Autodesk Inventor part; units mm, degrees
ref_plane "YZ Plane" through (0, 0, 0) normal (1, 0, 0) x (0, 1, 0)
ref_plane "XZ Plane" through (0, 0, 0) normal (0, 1, 0) x (-1, 0, 0)
ref_plane "XY Plane" through (0, 0, 0) normal (0, 0, 1) x (1, 0, 0)
sketch "Sketch1" plane through (0, 0, 0) normal (0, 0, 1) x (1, 0, 0)
  line L0 (-42.5, 5) -> (42.5, 5)
  line L1 (42.5, 5) -> (42.5, -5)
  line L2 (42.5, -5) -> (-42.5, -5)
  line L3 (-42.5, -5) -> (-42.5, 5)
  line L4 (-42.5, 5) -> (42.5, -5) construction
  line L5 (42.5, 5) -> (-42.5, -5) construction
  point P0 (0, 0)
  dimension "d0" = 85
  dimension "d1" = 10
extrude "Extrusion1" add sketch "Sketch1" along normal blind 0.5
sketch "Sketch2" plane through (0, 0, 0.5) normal (0, 0, 1) x (1, 0, 0)
  line L0 (-36.5, 2.5) -> (-31.5, 2.5)
  line L1 (-31.5, 2.5) -> (-31.5, -2.5)
  line L2 (-31.5, -2.5) -> (-36.5, -2.5)
  line L3 (-36.5, -2.5) -> (-36.5, 2.5)
  line L4 (-36.5, 2.5) -> (-31.5, -2.5) construction
  line L5 (-31.5, 2.5) -> (-36.5, -2.5) construction
  line L6 (-42.5, 5) -> (-42.5, -5)
  point P0 (0, 0)
  point P1 (-34, 0)
  point P2 (-34, 0)
  point P3 (-42.5, 0)
  dimension "d4" = 5
  dimension "d5" = 5
  dimension "d6" = 6
extrude "Extrusion2" add sketch "Sketch2" along normal blind 1.6
sketch "Sketch3" plane through (0, 0, 2.1) normal (0, 0, 1) x (1, 0, 0)
  line L0 (-31.5, 2.5) -> (-36.5, 2.5)
  line L1 (-36.5, 2.5) -> (-36.5, -2.5)
  line L2 (-36.5, -2.5) -> (-31.5, -2.5)
  line L3 (-31.5, -2.5) -> (-31.5, 2.5)
  circle A0 centre (-34, 0) radius 2.05
  point P0 (0, 0)
  point P1 (-31.5, 0)
  point P2 (-34, 2.5)
  dimension "d9" = 4.1
extrude "Extrusion3" cut sketch "Sketch3" against normal blind 0.1 contours A0
pattern_linear "Rectangular Pattern1" count 5 spacing 17 along (1, 0, 0) of "Extrusion3", "Extrusion2"
properties part number "LED Strip 5050 x 5"
Part model, mm, in its own coordinate system. A direction names the side the tool comes from. Give positions to 0.01 mm unless a question says otherwise; leave off trailing zeros. Write each loop counter-clockwise with the first axis right and the second up, starting at its lowest first coordinate (ties: lowest second). Pieces come first, ordered by that corner, then holes. Notation, with made-up numbers: (6.5, 5) -> (58.5, 5) arc R13 ccw to (58.5, 13) -> close; hole circle Ø2 at (62.5, 51.25). An arc over 180 degrees is marked (long way). Put each result on its own line as item: value. Start each with the question number.
Item 1: Cut at C-C (x = 4). List the corners of the cut face in (y, z).
Item 2: Pull direction X, two halves, no side cores. Call faces 1 (the face through (36.5, 0, 1)), 2 (the face through (-1, 0, 0)), 3 (the face through (0, 0, 2)): pulls with the +X half, pulls with the -X half, needs draft (parallel to the pull), parting line crosses it, or undercut.
Item 3: Which spindle directions (+Z, -Z, +X, -X, +Y, -Y) get a long thin tool onto all of the face, cutting with end or side? Do faces 4 (the face through (19.5, 0, 1)), 5 (the face through (0, -2.5, 1)), 6 (the face through (-34, 0, 2)), 7 (the face through (-17, 2.5, 1)). Say none if no direction does.
Item 4: Wall check: L1, parallel to Y at x = -35.5, z = 0.55; L2, parallel to Z at x = -27, y = 4.5; L3, parallel to Z at x = -33.5, y = 0. Give the ranges that are in metal, low to high. Write a range as [from, to].
Item 5: Pin check, flat tips, straight feed: pin 1 Ø0.5 at (y, z) = (0, 1.5) entering from +X; pin 2 Ø0.8 at (x, z) = (34.5, 1.5) entering from -Y; pin 3 Ø2 at (x, y) = (-33.5, -0.5) entering from +Z. Stop position of each tip, or through.
Item 6: Cut at A-A (x = -17). List the corners of the cut face in (y, z), then the cut area to 3 significant figures.
Item 7: Cut at B-B (y = 3.75). List the corners of the cut face in (x, z), then the cut area to 3 significant figures.
Answer list:
1. outline: (-5, 0) -> (5, 0) -> (5, 0.5) -> (-5, 0.5) -> close
2. face 1: pulls with the +X half
2. face 2: needs draft
2. face 3: undercut
3. face 4: +Z, +Y, -Y
3. face 5: +Z, +X, -X, -Y
3. face 6: +Z
3. face 7: +Z, +X, -X, +Y
4. L1: y = [-2.5, 2.5]
4. L2: z = [0, 0.5]
4. L3: z = [0, 2]
5. pin 1: stops at x = 36.5
5. pin 2: stops at y = -2.5
5. pin 3: stops at z = 2
6. outline: (-5, 0) -> (5, 0) -> (5, 0.5) -> (2.5, 0.5) -> (2.5, 2.1) -> (2.05, 2.1) -> (2.05, 2) -> (-2.05, 2) -> (-2.05, 2.1) -> (-2.5, 2.1) -> (-2.5, 0.5) -> (-5, 0.5) -> close
6. area: 12.6 mm2
7. outline: (-42.5, 0) -> (42.5, 0) -> (42.5, 0.5) -> (-42.5, 0.5) -> close
7. area: 42.5 mm2
